Can you work these out from the model? Positions are in its coordinate system, mm. Face numbers are marked on the shaded views. A direction names the side the tool comes from. Coordinates: 2 decimals unless noted, no trailing zeros. Order: outer loops, then holes, each group sorted by start corner. A loop starts at its lowest first (then second) coordinate and runs counter-clockwise, first axis right, second up.
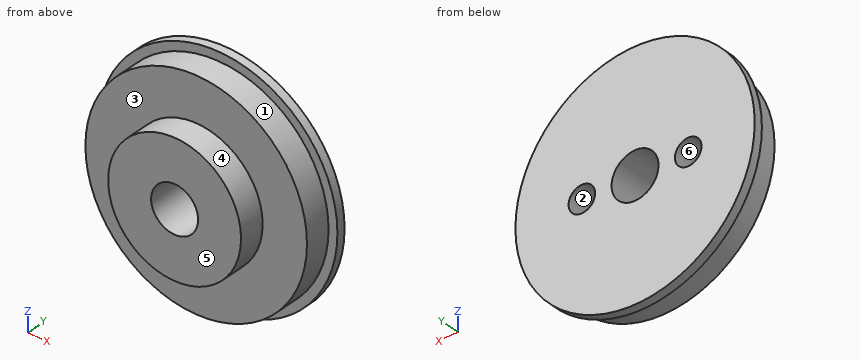
Autodesk Inventor part; units mm, degrees
ref_plane "YZ Plane" through (0, 0, 0) normal (1, 0, 0) x (0, 1, 0)
ref_plane "XZ Plane" through (0, 0, 0) normal (0, 1, 0) x (-1, 0, 0)
ref_plane "XY Plane" through (0, 0, 0) normal (0, 0, 1) x (1, 0, 0)
sketch "Szkic1" plane through (0, 0, 0) normal (0, 1, 0) x (-1, 0, 0)
  circle A0 centre (0, 0) radius 12.5
  dimension "d0" = 25
extrude "Wyciągnięcie proste1" add sketch "Szkic1" along normal blind 3
sketch "Szkic6" plane through (0, 3, 0) normal (0, 1, 0) x (1, 0, 0)
  circle A0 centre (0, 0) radius 13.5
  dimension "d13" = 27
extrude "Wyciągnięcie proste5" add sketch "Szkic6" along normal blind 1
sketch "Szkic7" plane through (0, 4, 0) normal (0, 1, 0) x (1, 0, 0)
  point P0 (0, 0)
  point P1 (-6, 0)
  dimension "d16" = 6
hole "Otwór1" at (-6, 4, 0) direction (0, -1, 0) diameter 3 depth 3
pattern_circular "Szyk kołowy1" count 2 over 360 about axis through (0, 3, 0) along (0, 1, 0) of "Otwór1"
sketch "Szkic8" plane through (0, 0, 0) normal (0, -1, 0) x (1, 0, 0)
  circle A0 centre (0, 0) radius 2.65
  dimension "d35" = 5.3
extrude "Wyciągnięcie proste6" cut sketch "Szkic8" against normal through all
sketch "Sketch10" plane through (0, 0, 0) normal (0, -1, 0) x (1, 0, 0)
  circle A0 centre (0, 0) radius 2.65
  circle A1 centre (0, 0) radius 7.5
  dimension "d36" = 15
extrude "Extrusion8" add sketch "Sketch10" along normal blind 3
properties part number "_Drukowanie 3D"
1. Imagine slicing it at B-B on z = 0. Please give me the cut outline in (x, y), then the cut area to 3 significant figures.
Completed:
outline: (-13.5, 3) - (-12.5, 3) - (-12.5, 0) - (-7.5, 0) - (-7.5, -3) - (-2.65, -3) - (-2.65, 4) - (-4.5, 4) - (-4.5, 1) - (-7.5, 1) - (-7.5, 4) - (-13.5, 4) - close; (2.65, -3) - (7.5, -3) - (7.5, 0) - (12.5, 0) - (12.5, 3) - (13.5, 3) - (13.5, 4) - (7.5, 4) - (7.5, 1) - (4.5, 1) - (4.5, 4) - (2.65, 4) - close
area: 91.9 mm2
2. Imagine slicing it at A-A on x = 0. Please give me the cut outline in (y, z), then the cut area to 3 significant figures.
Completed:
outline: (-3, -7.5) - (0, -7.5) - (0, -12.5) - (3, -12.5) - (3, -13.5) - (4, -13.5) - (4, -2.65) - (-3, -2.65) - close; (-3, 2.65) - (4, 2.65) - (4, 13.5) - (3, 13.5) - (3, 12.5) - (0, 12.5) - (0, 7.5) - (-3, 7.5) - close
area: 110 mm2
3. Imagine slicing it at D-D on y = 1.5. Please give me the cut outline in (x, z).
Completed:
outline: circle Ø25 at (0, 0); hole circle Ø3 at (-6, 0); hole circle Ø5.3 at (0, 0); hole circle Ø3 at (6, 0)
4. Thinking about a two-plate mould opening in X: for the marked faces 1, 2 and 3, which applies, pulls with the +X half, pulls with the -X half, needs draft (parallel to the pull), parting line crosses it, or undercut?
Completed:
face 1: parting line crosses it
face 2: undercut
face 3: needs draft
5. Imagine slicing it at C-C on y = -1. Please give me the cut outline in (x, z), then the cut area to 3 significant figures.
Completed:
outline: circle Ø15 at (0, 0); hole circle Ø5.3 at (0, 0)
area: 155 mm2
6. I'm going to push flat-ended pins straight in: pin 1 (1 mm diameter, centred on x = 10, y = -2, fed in from -Z); pin 2 (1.5 mm diameter, centred on x = 6.5, z = -0.5, fed in from +Y); pin 3 (3 mm diameter, centred on y = 3, z = 3, fed in from -X); pin 4 (1 mm diameter, centred on x = 9, y = 1.5, fed in from +Z). Where does each tip first touch, or does it pass through?
Completed:
pin 1: passes through
pin 2: stops at y = 1
pin 3: stops at x = -13.42
pin 4: stops at z = 9.17
7. Please list where these lines run through material, in increasing order: probe 1 along Z at (x, y) = (0, 1); probe 2 along Z at (x, y) = (0, -0.75); probe 3 along X at (y, z) = (-0.5, -6).
Completed:
probe 1: z = -12.5 to -2.65, 2.65 to 12.5
probe 2: z = -7.5 to -2.65, 2.65 to 7.5
probe 3: x = -4.5 to 4.5
8. On a 3-axis mill with a long thin cutter (end or side, diameter ignored), from which of +Z, -Z, +X, -X, +Y, -Y can I reach the whole of each face in a straight line? I mean the marked faces 4, 5 and 6. Say none if no direction works.
Completed:
face 4: -Y
face 5: +Z, -Z, +X, -X, -Y
face 6: +Y
